Source: CAD feature listing. Evaluate the final solid. Frame: model axes, mm. Give positions to 0.01 mm unless a question says otherwise; leave off trailing zeros. Order: outer loops, then holes, each group sorted by start corner. A loop starts at its lowest first (then second) coordinate and runs counter-clockwise, first axis right, second up. Notation, with made-up numbers: (-38, -3) -> (-2, -3) arc R21 ccw to (-2, 27) -> close; hole circle Ø3 at (85.5, 85). An arc over 180 degrees is marked (long way). Use CSV: the item, a comma, the result in double quotes.
```python
from build123d import *

# Parameters (mm, degrees)
BOSS_EXTRUDE1_DEPTH = 2.5
SKETCH2_R           = 1.5875
CUT_EXTRUDE1_DEPTH  = 15.145621231
CUT_EXTRUDE2_REACH  = 16.146
SKETCH5_R           = 0.665


with BuildPart() as part:
    # Sketch1 → Boss-Extrude1 (new, symmetric)
    with BuildSketch(Plane.XY):
        with BuildLine():
            Line((-8.94, 3.75), (8.94, 3.75))
            ThreePointArc((8.94, 3.75), (12.69, 0), (8.94, -3.75))
            Line((8.94, -3.75), (-8.94, -3.75))
            ThreePointArc((-8.94, -3.75), (-12.69, 0), (-8.94, 3.75))
        make_face()
    extrude(amount=BOSS_EXTRUDE1_DEPTH, both=True)

    # Sketch2 → Cut-Extrude1 (cut, through all)
    with BuildSketch(Plane.XY.offset(2.5)):
        with Locations((-8.94, 0)):
            Circle(SKETCH2_R)
        with Locations((8.94, 0)):
            Circle(SKETCH2_R)
    extrude(amount=-CUT_EXTRUDE1_DEPTH, mode=Mode.SUBTRACT)

    # Sketch5 → Cut-Extrude2 (cut, up to next)
    with BuildSketch(Plane.XY.offset(2.5), mode=Mode.PRIVATE) as cut_extrude2_sk1:
        with Locations((-4.49, 0)):
            Circle(SKETCH5_R)
    cut_extrude2_tool1 = extrude(cut_extrude2_sk1.sketch, amount=-CUT_EXTRUDE2_REACH, mode=Mode.PRIVATE) & part.part
    # Sketch5 → Cut-Extrude2 (cut, up to next)
    with BuildSketch(Plane.XY.offset(2.5), mode=Mode.PRIVATE) as cut_extrude2_sk2:
        with Locations((1.51, 0)):
            Circle(SKETCH5_R)
    cut_extrude2_tool2 = extrude(cut_extrude2_sk2.sketch, amount=-CUT_EXTRUDE2_REACH, mode=Mode.PRIVATE) & part.part
    add(cut_extrude2_tool1.solids().sort_by_distance((-4.49, 0, 2.5))[0], mode=Mode.SUBTRACT)
    add(cut_extrude2_tool2.solids().sort_by_distance((1.51, 0, 2.5))[0], mode=Mode.SUBTRACT)


solid = part.part
```
1. Section query B-B on z = 0.3. Count the separate pieces of the cut face and the enclosed holes in it, plus the area to 3 significant figures.
Answer below:
separate pieces,"1"
enclosed holes,"4"
area,"160 mm²"
2. Pin query (flat end, axial travel): P1, Ø3, axis at x = 8.94, y = 0, coming from the +Z side; P2, Ø1, axis at y = 2.5, z = 0, coming from the +X side. Return the tip coordinate at first contact, or that it passes through.
Answer below:
P1,"passes through"
P2,"stops at x = 12.11"
3. Mould query, pull axis X, two halves, no side actions, for faces 1 (the flat face through (0, 0, 2.5)), 2 (the cylindrical face through (-12.69, -0.08, 0.04)), 3 (the cylindrical face through (-3.876, -0.255, 0.035)). Classes: released by +X, released by -X, zero draft, split by the parting line, or undercut.
Answer below:
face 1,"zero draft"
face 2,"released by -X"
face 3,"undercut"
4. Section query A-A on y = 0. Return loops of the section in (x, z) (1 decimal).
Answer below:
outline,"(-12.7, -2.5) -> (-10.5, -2.5) -> (-10.5, 2.5) -> (-12.7, 2.5) -> close; (-7.4, -2.5) -> (-5.2, -2.5) -> (-5.2, 2.5) -> (-7.4, 2.5) -> close; (-3.8, -2.5) -> (0.8, -2.5) -> (0.8, 2.5) -> (-3.8, 2.5) -> close; (2.2, -2.5) -> (7.4, -2.5) -> (7.4, 2.5) -> (2.2, 2.5) -> close; (10.5, -2.5) -> (12.7, -2.5) -> (12.7, 2.5) -> (10.5, 2.5) -> close"
5. Section query D-D on y = -1. Return loops of the section in (x, z), plus the area to 3 significant figures.
Answer below:
outline,"(-12.55, -2.5) -> (-10.17, -2.5) -> (-10.17, 2.5) -> (-12.55, 2.5) -> close; (-7.71, -2.5) -> (7.71, -2.5) -> (7.71, 2.5) -> (-7.71, 2.5) -> close; (10.17, -2.5) -> (12.55, -2.5) -> (12.55, 2.5) -> (10.17, 2.5) -> close"
area,"101 mm²"
6. Ray query, line 1 along Y through (x, z) = (1.51, -0.6) (3 decimals); line 2 along X through (y, z) = (1, 1.6); line 3 along Y through (x, z) = (8.94, -0.05). Return the intervals inside material, ascending.
Answer below:
line 1,"y = -3.75 to -0.665, 0.665 to 3.75"
line 2,"x = -12.55 to -10.17, -7.71 to 7.71, 10.17 to 12.55"
line 3,"y = -3.75 to -1.59, 1.59 to 3.75"
7. Section query C-C on x = 1.51. Return loops of the section in (y, z) (3 decimals), plus the area to 4 significant figures.
Answer below:
outline,"(-3.75, -2.5) -> (-0.665, -2.5) -> (-0.665, 2.5) -> (-3.75, 2.5) -> close; (0.665, -2.5) -> (3.75, -2.5) -> (3.75, 2.5) -> (0.665, 2.5) -> close"
area,"30.85 mm²"
